Part model, mm, in its own coordinate system. Face numbers are marked on the shaded views. A direction names the side the tool comes from. Give positions to 0.01 mm unless a question says otherwise; leave off trailing zeros. Write each loop counter-clockwise with the first axis right and the second up, starting at its lowest first coordinate (ties: lowest second). Pieces come first, ordered by that corner, then holes.
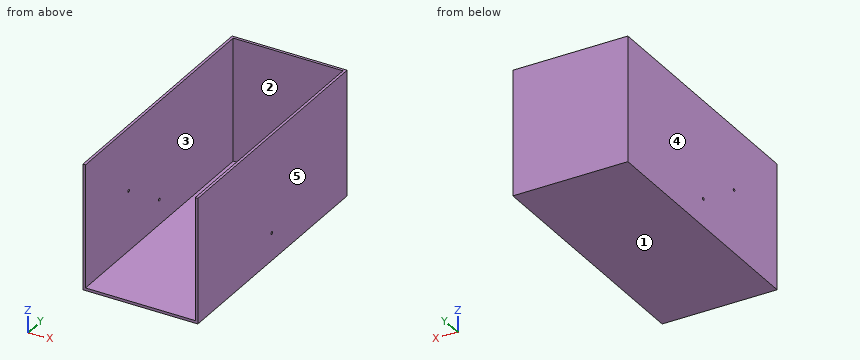
from build123d import *

# Parameters (mm, degrees)
F0_W     = 266.7
F0_H     = 609.4600376606
F1_DEPTH = 6.35
F2_DEPTH = 304.8
F3_R     = 3.302
F4_DEPTH = 279.401
F5_R     = 3.302
F6_DEPTH = 25.4


with BuildPart() as f1:
    # F0 (on Top) → F1 (new body)
    with BuildSketch(Plane.XY):
        with Locations((0, 0.0699811697)):
            Rectangle(F0_W, F0_H)
    extrude(amount=F1_DEPTH)

    # F0 (on Top) → F2 (join)
    with BuildSketch(Plane.XY):
        Polygon((-133.35, 304.8), (133.35, 304.8), (133.35, -304.6600376606), (139.7, -304.6600376606), (139.7, 311.15), (-139.7, 311.15), (-139.7, -304.6600376606), (-133.35, -304.6600376606), align=None)
    extrude(amount=F2_DEPTH)

    # F3 (on face) → F4 (cut, through all)
    with BuildSketch(Plane.YZ.offset(139.7)):
        with Locations((0, 66.802)):
            Circle(F3_R)
    extrude(amount=-F4_DEPTH, mode=Mode.SUBTRACT)

    # F5 (on face) → F6 (cut)
    with BuildSketch(Plane.YZ.offset(-133.35)):
        with Locations((-126.8600376606, 152.4)):
            Circle(F5_R)
    extrude(amount=-F6_DEPTH, mode=Mode.SUBTRACT)


solid = f1.part
1) Drill centre lines: L1, parallel to Y at x = -136.5, z = 152.4; L2, parallel to X at y = 118.5, z = 235.5; L3, parallel to Z at x = -135, y = 0. Where is each one in solid material? Low to high.
Check result:
L1: y = -304.66 to -130.16, -123.56 to 311.15
L2: x = -139.7 to -133.35, 133.35 to 139.7
L3: z = 0 to 63.5, 70.1 to 304.8
2) Saw through at A-A (z = 176). Write the cut outline in (x, y).
Check result:
outline: (-139.7, -304.66) - (-133.35, -304.66) - (-133.35, 304.8) - (133.35, 304.8) - (133.35, -304.66) - (139.7, -304.66) - (139.7, 311.15) - (-139.7, 311.15) - close
3) Mould opens along X. For the marked faces 3, 4 and 5 say: +X half, -X half, draft (parallel to the pull), parting line (faces both ways), or undercut.
Check result:
face 3: undercut
face 4: -X half
face 5: +X half
4) Saw through at B-B (y = 231.5). Write the cut outline in (x, z), and give its area (3 significant figures).
Check result:
outline: (-139.7, 0) - (139.7, 0) - (139.7, 304.8) - (133.35, 304.8) - (133.35, 6.35) - (-133.35, 6.35) - (-133.35, 304.8) - (-139.7, 304.8) - close
area: 5,560 mm2
5) Flat gauge pins, fed straight in: P1, Ø7.5, axis at y = 0, z = 66.802, coming from the -X side; P2, Ø12, axis at x = 5, y = 9.5, coming from the +Z side; P3, Ø12, axis at x = 40.5, z = 138, coming from the -Y side. Where does each tip first touch, or does it go through?
Check result:
P1: stops at x = -139.7
P2: stops at z = 6.35
P3: stops at y = 304.8
6) Saw through at C-C (x = 22.5). Write the cut outline in (y, z), and give its area (3 significant figures).
Check result:
outline: (-304.66, 0) - (311.15, 0) - (311.15, 304.8) - (304.8, 304.8) - (304.8, 6.35) - (-304.66, 6.35) - close
area: 5,810 mm2
7) 3-axis set-ups, long thin cutter, end or side, ignore diameter. For the marked faces 1 and 2: which of +Z, -Z, +X, -X, +Y, -Y reach the whole face in a straight line?
Check result:
face 1: -Z, +X, -X, +Y, -Y
face 2: +Z, -Y
